Work out the finished part from the listing and answer in its coordinate system (mm). A direction names the side the tool comes from. Give positions to 0.01 mm unless a question says otherwise; leave off trailing zeros. Order: outer loops, then holes, each group sorted by start corner. A loop starts at its lowest first (then second) coordinate and runs counter-clockwise, first axis right, second up. Notation, with made-up numbers: (-6, 17.5) - (34, 17.5) arc R28 cw to (34, 37.5) - close; hole circle Ø4 at (57.25, -13). An arc over 180 degrees is marked (long way). Put each result on its own line as item: value.
```python
from build123d import *

# Parameters (mm, degrees)
SKETCH_1_W          = 20
SKETCH_1_H          = 20
SKETCH_1_W_2        = 16
SKETCH_1_H_2        = 16
EXTRUDE_1_DEPTH     = 250
SKETCH_2_R          = 1.6
CUT_EXTRUDE_1_DEPTH = 252.594912508
SKETCH_3_R          = 1.6
CUT_EXTRUDE_2_DEPTH = 252.594912508
SKETCH_4_R          = 1.6
CUT_EXTRUDE_3_DEPTH = 252.594912508
SKETCH_5_R          = 1.6
CUT_EXTRUDE_4_DEPTH = 252.594912508


with BuildPart() as part:
    # 草图1 → 拉伸-薄壁1 (new body)
    with BuildSketch(Plane.XY):
        with Locations((10, 10)):
            Rectangle(SKETCH_1_W, SKETCH_1_H)
        with Locations((10, 10)):
            Rectangle(SKETCH_1_W_2, SKETCH_1_H_2, mode=Mode.SUBTRACT)
    extrude(amount=EXTRUDE_1_DEPTH)

    # 草图2 → 切除-拉伸1 (cut, through all)
    with BuildSketch(Plane.XZ):
        with Locations(Location((10, 10, 0), (0, 0, 270))):
            Circle(SKETCH_2_R)
        with Locations(Location((10, 30, 0), (0, 0, 270))):
            Circle(SKETCH_2_R)
        with Locations(Location((10, 50, 0), (0, 0, 270))):
            Circle(SKETCH_2_R)
    extrude(amount=-CUT_EXTRUDE_1_DEPTH, mode=Mode.SUBTRACT)

    # 草图3 → 切除-拉伸2 (cut, through all)
    with BuildSketch(Plane(origin=(0, 20, 0), x_dir=(1, 0, 0), z_dir=(0, 1, 0))):
        with Locations(Location((10, -150, 0), (0, 0, 270))):
            Circle(SKETCH_3_R)
        with Locations(Location((10, -170, 0), (0, 0, 270))):
            Circle(SKETCH_3_R)
        with Locations(Location((10, -190, 0), (0, 0, 270))):
            Circle(SKETCH_3_R)
        with Locations(Location((10, -245, 0), (0, 0, 270))):
            Circle(SKETCH_3_R)
        with Locations(Location((10, -225, 0), (0, 0, 270))):
            Circle(SKETCH_3_R)
    extrude(amount=-CUT_EXTRUDE_2_DEPTH, mode=Mode.SUBTRACT)

    # 草图4 → 切除-拉伸3 (cut, through all)
    with BuildSketch(Plane(origin=(20, 0, 0), x_dir=(0, 0, -1), z_dir=(1, 0, 0))):
        with Locations((-230, 10)):
            Circle(SKETCH_4_R)
        with Locations((-190, 10)):
            Circle(SKETCH_4_R)
    extrude(amount=-CUT_EXTRUDE_3_DEPTH, mode=Mode.SUBTRACT)

    # 草图5 → 切除-拉伸4 (cut, through all)
    with BuildSketch(Plane(origin=(20, 0, 0), x_dir=(0, 0, -1), z_dir=(1, 0, 0))):
        with Locations((-90, 10)):
            Circle(SKETCH_5_R)
        with Locations((-115, 10)):
            Circle(SKETCH_5_R)
        with Locations((-65, 10)):
            Circle(SKETCH_5_R)
    extrude(amount=-CUT_EXTRUDE_4_DEPTH, mode=Mode.SUBTRACT)


solid = part.part
```
(1) Section B-B, the plane y = 15.5 is taken. Write down the section's boundary in (x, z).
Geometry check:
outline: (0, 0) - (2, 0) - (2, 250) - (0, 250) - close; (18, 0) - (20, 0) - (20, 250) - (18, 250) - close
(2) A tool of negligible diameter and unlimited length cuts with its end or side. For faces 5 (the face through (1, 10, 0)), 6 (the face through (2, 10, 123)), from which of +Z, -Z, +X, -X, +Y, -Y can it reach the whole face along a straight path? Write none if from no direction.
Geometry check:
face 5: -Z, +X, -X, +Y, -Y
face 6: +Z, -Z
(3) Determine the mould class of faces 1 (the face through (10, 2, 123)), 2 (the face through (10, 20, 123)), 3 (the face through (18, 10, 123)), 4 (the face through (0, 10, 123)) for opening direction Y: pulls with the +Y half, pulls with the -Y half, needs draft (parallel to the pull), parting line crosses it, or undercut.
Geometry check:
face 1: undercut
face 2: pulls with the +Y half
face 3: undercut
face 4: needs draft
(4) Section A-A, the plane z = 42 is taken. Write down the section's boundary in (x, y), then the cut area to 3 significant figures.
Geometry check:
outline: (0, 0) - (20, 0) - (20, 20) - (0, 20) - close; hole (2, 2) - (18, 2) - (18, 18) - (2, 18) - close
area: 144 mm²
(5) Straight lines are drawn through the part: line 1 (Y direction, x = 19.55, z = 190); line 2 (Y direction, x = 6, z = 227.5). For each, find the intervals that lie inside material, in ascending order.
Geometry check:
line 1: y = 0 to 8.4, 11.6 to 20
line 2: y = 0 to 2, 18 to 20
(6) Given pin 1 (5 mm diameter, centred on y = 10, z = 65, fed in from -X), flat-ended and moving along its own axis, determine where the tip first touches the part or whether it passes through.
Geometry check:
pin 1: stops at x = 0
